Model file for the job. Use its own axes, mm. A direction names the side the tool comes from. Round coordinates to 2 decimals unless told otherwise and drop trailing zeros. Loops run counter-clockwise (first coordinate to the right, second up) from the corner with the lowest first, then second, coordinate; pieces in that order, holes last. Notation, with made-up numbers: M 70,19 L 129,19 A28 cw 129,49 Z; hole C 0.25,13.25 d2. An arc over 180 degrees is marked long. Use a Markdown table: item, result. Add a question column.
Q1. Tool access for faces 4 (the face through (6, 76.2, 6)), 5 (the face through (6, 50.8, 6)), 6 (the face through (527, 76.2, 6)), 7 (the face through (527, 38.1, 6)): list every direction of +Z, -Z, +X, -X, +Y, -Y with a clear straight run to the whole face (end or side of a thin tool).
Q2. Pin check, flat tips, straight feed: pin 1 (1.5 mm diameter, centred on y = 37, z = 7.5, fed in from +X); pin 2 (4 mm diameter, centred on x = 525, z = 8.5, fed in from +Y); pin 3 (4 mm diameter, centred on x = 525.5, z = 9.5, fed in from -Y). Stop position of each tip, or through.
Q3. Cut at A-A (z = 6.5). Give the cut face in (x, y), plus the area to 3 significant figures.
Q4. Cut at B-B (y = 32.5). Give the cut face in (x, z).
Q5. Probe line 1 (X direction, y = 6.5, z = 1). List the from-to ranges inside material, lowest first. Write a range as from..to.
Q6. Mould opens along Y. For faces 1 (the face through (527, 63.5, 6)), 2 (the face through (6, 12.7, 6)), 3 (the face through (0, 70, 6)) say: +Y half, -Y half, draft (parallel to the pull), parting line (faces both ways), or undercut.
from build123d import *

# Parameters (mm, degrees)
F0_W     = 533.4
F0_H     = 88.9
F1_DEPTH = 12.7
F2_W     = 12.7
F2_H     = 12.7
F3_DEPTH = 25.4
F4_W     = 12.7
F4_H     = 12.7
F5_DEPTH = 25.4


with BuildPart() as f1:
    # F0 (on Top) → F1 (new body)
    with BuildSketch(Plane.XY):
        with Locations((266.7, 44.45)):
            Rectangle(F0_W, F0_H)
    extrude(amount=F1_DEPTH)

    # F2 (on face) → F3 (cut)
    with BuildSketch(Plane.XY.offset(12.7)):
        with Locations((527.05, 6.35)):
            Rectangle(F2_W, F2_H)
        with Locations((527.05, 31.75)):
            Rectangle(F2_W, F2_H)
        with Locations((527.05, 57.15)):
            Rectangle(F2_W, F2_H)
        with Locations((527.05, 82.55)):
            Rectangle(F2_W, F2_H)
    extrude(amount=-F3_DEPTH, mode=Mode.SUBTRACT)

    # F4 (on face) → F5 (cut)
    with BuildSketch(Plane.XY.offset(12.7)):
        with Locations((6.35, 6.35)):
            Rectangle(F4_W, F4_H)
        with Locations((6.35, 31.75)):
            Rectangle(F4_W, F4_H)
        with Locations((6.35, 82.55)):
            Rectangle(F4_W, F4_H)
        with Locations((6.35, 57.15)):
            Rectangle(F4_W, F4_H)
    extrude(amount=-F5_DEPTH, mode=Mode.SUBTRACT)


solid = f1.part
Checked values:
| question | item | result |
|---|---|---|
| 1 | face 4 | +Z, -Z, -X, +Y |
| 1 | face 5 | +Z, -Z, -X |
| 1 | face 6 | +Z, -Z, +X, +Y |
| 1 | face 7 | +Z, -Z, +X |
| 2 | pin 1 | stops at x = 520.7 |
| 2 | pin 2 | stops at y = 76.2 |
| 2 | pin 3 | stops at y = 12.7 |
| 3 | outline | M 0,12.7 L 12.7,12.7 L 12.7,0 L 520.7,0 L 520.7,12.7 L 533.4,12.7 L 533.4,25.4 L 520.7,25.4 L 520.7,38.1 L 533.4,38.1 L 533.4,50.8 L 520.7,50.8 L 520.7,63.5 L 533.4,63.5 L 533.4,76.2 L 520.7,76.2 L 520.7,88.9 L 12.7,88.9 L 12.7,76.2 L 0,76.2 L 0,63.5 L 12.7,63.5 L 12.7,50.8 L 0,50.8 L 0,38.1 L 12.7,38.1 L 12.7,25.4 L 0,25.4 Z |
| 3 | area | 46,100 mm^2 |
| 4 | outline | M 12.7,0 L 520.7,0 L 520.7,12.7 L 12.7,12.7 Z |
| 5 | line 1 | x = 12.7..520.7 |
| 6 | face 1 | undercut |
| 6 | face 2 | -Y half |
| 6 | face 3 | draft |
